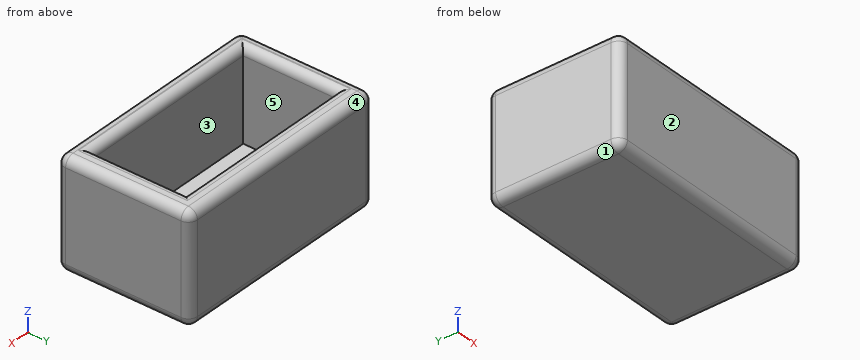
from build123d import *

# Parameters (mm, degrees)
BOX038_W     = 20.3
BOX038_H     = 10.3
BOX038_DEPTH = 300
BOX039_W     = 24.8
BOX039_H     = 14.8
BOX039_DEPTH = 12
FILLET019_R  = 1
FILLET020_R  = 0.9


with BuildPart() as cube_20x10_clone001:
    # Box038 → Box038 (new body)
    with BuildSketch(Plane.XY):
        with Locations((10.15, 5.15)):
            Rectangle(BOX038_W, BOX038_H)
    extrude(amount=BOX038_DEPTH)


with BuildPart() as cube_20x10_clone001_1:
    # Body012 placement: moved
    add(cube_20x10_clone001.part.moved(Location((2, 2, 2))))


with BuildPart() as profile_cap_outer_fillet:
    # Box039 → Box039 (new body)
    with BuildSketch(Plane.XY):
        with Locations((12.4, 7.4)):
            Rectangle(BOX039_W, BOX039_H)
    extrude(amount=BOX039_DEPTH)

    # Fillet019
    fillet019_edges = [profile_cap_outer_fillet.edges().sort_by_distance(p)[0] for p in [
        (0, 0, 6),
        (0, 7.4, 12),
        (0, 14.8, 6),
        (0, 7.4, 0),
        (24.8, 0, 6),
        (24.8, 7.4, 12),
        (24.8, 14.8, 6),
        (24.8, 7.4, 0),
        (12.4, 0, 0),
        (12.4, 0, 12),
        (12.4, 14.8, 0),
        (12.4, 14.8, 12),
    ]]
    fillet(fillet019_edges, radius=FILLET019_R)

    # Cut023012: cut cube 20x10 clone001
    add(cube_20x10_clone001_1.part, mode=Mode.SUBTRACT)

    # Fillet020
    fillet020_edges = [profile_cap_outer_fillet.edges().sort_by_distance(p)[0] for p in [
        (12.15, 2, 12),
        (22.3, 7.15, 12),
        (12.15, 12.3, 12),
        (2, 7.15, 12),
    ]]
    fillet(fillet020_edges, radius=FILLET020_R)


solid = profile_cap_outer_fillet.part
Check sheet for the modelled part. Datum: model origin and axes. Units: mm. Face numbers are marked on the shaded views. A direction names the side the tool comes from. Coordinates: 2 decimals unless noted, no trailing zeros. Loops run counter-clockwise (first coordinate to the right, second up) from the corner with the lowest first, then second, coordinate; pieces in that order, holes last. Notation, with made-up numbers: (-7, 86) -> (52, 86) arc R21 ccw to (52, 113) -> close; hole circle Ø11 at (62.25, -11.75). An arc over 180 degrees is marked (long way). Write item = value, one per line. Start each with the question number.
1. Draft check along Y on the marked faces 1, 2 and 3. Enter one of: released by +Y, released by -Y, zero draft, split by the parting line, or undercut.
2. Section check A-A on y = 4. Record the cut outline in (x, z), then the cut area to 3 significant figures.
3. Section check C-C on x = 20.75. Record the cut outline in (y, z), then the cut area to 3 significant figures.
4. Material ranges on line 1 (X direction, y = 2.75, z = 5.25); line 2 (Y direction, x = 9.25, z = 7); line 3 (Y direction, x = 14, z = 11.5), recorded low to high.
5. Tool access check on the marked faces 4 and 5. Record the directions out of +Z, -Z, +X, -X, +Y, -Y that give a thin tool (end or side, any length) a straight path to the whole face; none if there is none.
6. Depth check by flat-ended pin: P1, Ø6, axis at x = 10.5, y = 4.5, coming from the -Z side; P2, Ø3, axis at x = 13, y = 5.5, coming from the +Z side. Enter the tip coordinate at first touch or a pass-through.
7. Section check B-B on z = 3.75. Record the cut outline in (x, y).
Responses:
q1.face_1 = zero draft
q1.face_2 = released by -Y
q1.face_3 = undercut
q2.outline = (0, 1) arc R1 ccw to (1, 0) -> (23.8, 0) arc R1 ccw to (24.8, 1) -> (24.8, 11) arc R1 ccw to (23.8, 12) -> (23.2, 12) arc R0.9 ccw to (22.3, 11.1) -> (22.3, 2) -> (2, 2) -> (2, 11.1) arc R0.9 ccw to (1.1, 12) -> (1, 12) arc R1 ccw to (0, 11) -> close
q2.area = 93.4 mm2
q3.outline = (0, 1) arc R1 ccw to (1, 0) -> (13.8, 0) arc R1 ccw to (14.8, 1) -> (14.8, 11) arc R1 ccw to (13.8, 12) -> (13.2, 12) arc R0.9 ccw to (12.3, 11.1) -> (12.3, 2) -> (2, 2) -> (2, 11.1) arc R0.9 ccw to (1.1, 12) -> (1, 12) arc R1 ccw to (0, 11) -> close
q3.area = 73.4 mm2
q4.line_1 = 0 to 2, 22.3 to 24.8
q4.line_2 = 0 to 2, 12.3 to 14.8
q4.line_3 = 0.13 to 1.91, 12.39 to 14.67
q5.face_4 = +Z, +X, -X, +Y
q5.face_5 = +Z
q6.P1 = 0
q6.P2 = 2
q7.outline = (0, 1) arc R1 ccw to (1, 0) -> (23.8, 0) arc R1 ccw to (24.8, 1) -> (24.8, 13.8) arc R1 ccw to (23.8, 14.8) -> (1, 14.8) arc R1 ccw to (0, 13.8) -> close; hole (2, 2) -> (22.3, 2) -> (22.3, 12.3) -> (2, 12.3) -> close
